```python
from build123d import *

# Parameters (mm, degrees)
SZKIC1_W                    = 76
SZKIC1_H                    = 16.4
SZKIC1_R                    = 2
DODANIE_WYCI_GNI_CIE1_DEPTH = 1.6
SZKIC2_W                    = 6
SZKIC2_H                    = 6
DODANIE_WYCI_GNI_CIE2_DEPTH = 3
SZKIC3_R                    = 1.75
DODANIE_WYCI_GNI_CIE3_DEPTH = 1
SZKIC4_R                    = 1.5
DODANIE_WYCI_GNI_CIE4_DEPTH = 6
ZAOKR_GLENIE1_R             = 1.5
SZKIC5_W                    = 22
SZKIC5_H                    = 6
DODANIE_WYCI_GNI_CIE5_DEPTH = 4.5


with BuildPart() as part:
    # Szkic1 → Dodanie-wyciągnięcie1 (new body)
    with BuildSketch(Plane(origin=(0, 0, 0), x_dir=(1, 0, 0), z_dir=(0, 1, 0))):
        Rectangle(SZKIC1_W, SZKIC1_H)
        with Locations((-22.9, -3.2)):
            Circle(SZKIC1_R, mode=Mode.SUBTRACT)
        with Locations((22.5, -3.2)):
            Circle(SZKIC1_R, mode=Mode.SUBTRACT)
    extrude(amount=DODANIE_WYCI_GNI_CIE1_DEPTH)

    # Szkic2 → Dodanie-wyciągnięcie2 (add)
    with BuildSketch(Plane(origin=(0, 1.6, 0), x_dir=(1, 0, 0), z_dir=(0, 1, 0))):
        with Locations((-32, -3.6)):
            Rectangle(SZKIC2_W, SZKIC2_H)
        with Locations((-13.4, -3.6)):
            Rectangle(SZKIC2_W, SZKIC2_H)
        with Locations((-1, -3.6)):
            Rectangle(SZKIC2_W, SZKIC2_H)
        with Locations((14.7, -3.6)):
            Rectangle(SZKIC2_W, SZKIC2_H)
        with Locations((32.5, -3.6)):
            Rectangle(SZKIC2_W, SZKIC2_H)
    extrude(amount=DODANIE_WYCI_GNI_CIE2_DEPTH)

    # Szkic3 → Dodanie-wyciągnięcie3 (add)
    with BuildSketch(Plane(origin=(0, 4.6, 0), x_dir=(1, 0, 0), z_dir=(0, 1, 0))):
        with Locations((-32, -3.6)):
            Circle(SZKIC3_R)
        with Locations((-13.4, -3.6)):
            Circle(SZKIC3_R)
        with Locations((-1, -3.6)):
            Circle(SZKIC3_R)
        with Locations((14.7, -3.6)):
            Circle(SZKIC3_R)
        with Locations((32.5, -3.6)):
            Circle(SZKIC3_R)
    extrude(amount=DODANIE_WYCI_GNI_CIE3_DEPTH)

    # Szkic4 → Dodanie-wyciągnięcie4 (add)
    with BuildSketch(Plane(origin=(0, 1.6, 0), x_dir=(1, 0, 0), z_dir=(0, 1, 0))):
        with Locations((-33.5, 4.2)):
            Circle(SZKIC4_R)
    extrude(amount=DODANIE_WYCI_GNI_CIE4_DEPTH)

    # Zaokrąglenie1
    zaokr_glenie1_edges = [part.edges().sort_by_distance(p)[0] for p in [
        (-35, 7.6, -4.2),
    ]]
    fillet(zaokr_glenie1_edges, radius=ZAOKR_GLENIE1_R)

    # Szkic5 → Dodanie-wyciągnięcie5 (add)
    with BuildSketch(Plane(origin=(0, 1.6, 0), x_dir=(1, 0, 0), z_dir=(0, 1, 0))):
        with Locations((-16, 6.2)):
            Rectangle(SZKIC5_W, SZKIC5_H)
    extrude(amount=DODANIE_WYCI_GNI_CIE5_DEPTH)


solid = part.part
```
Check sheet for the modelled part. Datum: model origin and axes. Units: mm. A direction names the side the tool comes from. Round coordinates to 2 decimals unless told otherwise and drop trailing zeros. Loops run counter-clockwise (first coordinate to the right, second up) from the corner with the lowest first, then second, coordinate; pieces in that order, holes last. Notation, with made-up numbers: (50, 85.25) - (92, 85.25) arc R26 ccw to (92, 122.25) - close; hole circle Ø6 at (40.25, 89.25). An arc over 180 degrees is marked (long way). Answer as a JSON object with one key per item and string values. Group by question number.
Q1. Gauge pin test, flat ends, axial feed: P1, Ø3.5, axis at y = 3.5, z = 4, coming from the +X side; P2, Ø3.5, axis at x = 31.5, y = 3.5, coming from the +Z side; P3, Ø3, axis at x = -12, z = 2.5, coming from the +Y side; P4, Ø2.5, axis at y = 2.5, z = 3, coming from the +X side. Record the tip position at first contact, or that the pin passes through.
Q2. Sectioned sample at C-C, the plane x = 32.5. Enter the section's corners in (y, z).
Q3. Set-up check for faces 4 (the face through (-34.7, 3.8, -3.3)), 5 (the face through (-16, 6.1, -6)), 6 (the face through (17.7, 3, 4)): record each of +Z, -Z, +X, -X, +Y, -Y from which the full face is reachable in a straight line by a thin tool's end or side.
Q4. Sectioned sample at A-A, the plane x = -22.9. Enter the section's corners in (y, z), plus the area to 3 significant figures.
Q5. Mould release check, pull along X, two halves, no side actions. Record for faces 1 (the face through (2, 3, 4)), 2 (the face through (-35, 3, 4)), 3 (the face through (15, 3, 6.6)): released by +X, released by -X, zero draft, split by the parting line, or undercut.
Q6. Sectioned sample at B-B, the plane z = -4.2. Enter the section's corners in (x, y), plus the area to 3 significant figures.
Q7. Scan lines: line 1 along X through (y, z) = (0.8, 3.2); line 2 along Z through (x, y) = (-22.9, 0.55); line 3 along Y through (x, z) = (-5.5, 0). Record each from-to range of solid material in increasing order. Write a range as [from, to].
Q8. Sectioned sample at D-D, the plane x = 22.5. Enter the section's corners in (y, z), plus the area to 3 significant figures.
Solution:
{
 "1": {"P1": "stops at x = 35.5", "P2": "stops at z = 6.6", "P3": "stops at y = 5.6", "P4": "stops at x = 38"},
 "2": {"outline": "(0, -8.2) - (1.6, -8.2) - (1.6, 0.6) - (4.6, 0.6) - (4.6, 1.85) - (5.6, 1.85) - (5.6, 5.35) - (4.6, 5.35) - (4.6, 6.6) - (1.6, 6.6) - (1.6, 8.2) - (0, 8.2) - close"},
 "3": {"face 4": "+Y", "face 5": "+Z, -Z, +X, +Y", "face 6": "+Z, -Z, +Y"},
 "4": {"outline": "(0, -8.2) - (1.6, -8.2) - (1.6, -9.2) - (6.1, -9.2) - (6.1, -3.2) - (1.6, -3.2) - (1.6, 1.2) - (0, 1.2) - close; (0, 5.2) - (1.6, 5.2) - (1.6, 8.2) - (0, 8.2) - close", "area": "46.8 mm²"},
 "5": {"face 1": "undercut", "face 2": "released by -X", "face 3": "zero draft"},
 "6": {"outline": "(-38, 0) - (38, 0) - (38, 1.6) - (-5, 1.6) - (-5, 6.1) - (-27, 6.1) - (-27, 1.6) - (-32, 1.6) - (-32, 6.1) arc R1.5 ccw to (-35, 6.1) - (-35, 1.6) - (-38, 1.6) - close", "area": "238 mm²"},
 "7": {"line 1": "x = [-38, -24.9], [-20.9, 20.5], [24.5, 38]", "line 2": "z = [-8.2, 1.2], [5.2, 8.2]", "line 3": "y = [0, 1.6]"},
 "8": {"outline": "(0, -8.2) - (1.6, -8.2) - (1.6, 1.2) - (0, 1.2) - close; (0, 5.2) - (1.6, 5.2) - (1.6, 8.2) - (0, 8.2) - close", "area": "19.8 mm²"}
}
